```python
from build123d import *

# Parameters (mm, degrees)
SKETCH1_R           = 3.429
SKETCH1_R_2         = 2.54
BOSS_EXTRUDE1_DEPTH = 3.2004
SKETCH2_R           = 1.7272
CUT_EXTRUDE1_DEPTH  = 3.2004
SKETCH5_R           = 1.7272
SKETCH5_W           = 40.894
SKETCH5_H           = 20.32
CUT_EXTRUDE3_DEPTH  = 4.2004
CUT_EXTRUDE4_DEPTH  = 3.2004
SKETCH8_R           = 1.7272
CUT_EXTRUDE6_DEPTH  = 3.2004
SKETCH9_R           = 2.54
CUT_EXTRUDE7_DEPTH  = 3.2004
CUT_EXTRUDE8_DEPTH  = 3.2004
FILLET1_R           = 5.08
SKETCH12_R          = 2.159
CUT_EXTRUDE10_DEPTH = 3.2004
SKETCH13_R          = 13.885201093
CUT_EXTRUDE11_DEPTH = 3.2004
SKETCH14_R          = 3.175
CUT_EXTRUDE12_DEPTH = 3.2004


with BuildPart() as part:
    # Sketch1 → Boss-Extrude1 (new body)
    with BuildSketch(Plane.XY):
        with BuildLine():
            Line((0, 0), (120.015, 0))
            ThreePointArc((120.015, 0), (130.351788396, 3.075697789), (137.325636158, 11.302152592))
            Line((137.325636158, 11.302152592), (155.2575, 52.11572))
            ThreePointArc((155.2575, 52.11572), (157.086103359, 70.33575546), (147.862829498, 86.154880014))
            ThreePointArc((147.862829498, 86.154880014), (60.0075, 119.675648405), (-27.847829498, 86.154880014))
            ThreePointArc((-27.847829498, 86.154880014), (-37.071103359, 70.33575546), (-35.2425, 52.11572))
            Line((-35.2425, 52.11572), (-17.310636158, 11.302152592))
            ThreePointArc((-17.310636158, 11.302152592), (-10.336788396, 3.075697789), (0, 0))
        make_face()
        with Locations((120.015, 18.90776)):
            Circle(SKETCH1_R, mode=Mode.SUBTRACT)
        with Locations((0, 18.90776)):
            Circle(SKETCH1_R, mode=Mode.SUBTRACT)
        with Locations((19.734727639, 25.566426996)):
            Circle(SKETCH1_R_2, mode=Mode.SUBTRACT)
    extrude(amount=BOSS_EXTRUDE1_DEPTH)

    # Sketch2 → Cut-Extrude1 (cut)
    with BuildSketch(Plane(origin=(0, 0, 0), x_dir=(-1, 0, 0), z_dir=(0, 0, -1))):
        with Locations((-92.0115, 52.11572)):
            Circle(SKETCH2_R)
        with Locations((-76.0095, 52.11572)):
            Circle(SKETCH2_R)
        with Locations((-44.0055, 52.11572)):
            Circle(SKETCH2_R)
        with Locations((-28.0035, 52.11572)):
            Circle(SKETCH2_R)
    extrude(amount=-CUT_EXTRUDE1_DEPTH, mode=Mode.SUBTRACT)

    # Sketch5 → Cut-Extrude3 (cut, through all)
    with BuildSketch(Plane(origin=(0, 0, 0), x_dir=(-1, 0, 0), z_dir=(0, 0, -1))):
        with Locations((-79.746999972, 23.90776)):
            Circle(SKETCH5_R)
        with Locations((-29.246999972, 13.90776)):
            Circle(SKETCH5_R)
        with Locations((-29.246999972, 23.90776)):
            Circle(SKETCH5_R)
        with Locations((-79.746999972, 13.90776)):
            Circle(SKETCH5_R)
        with Locations((-92.322240346, 23.90776)):
            Circle(SKETCH5_R)
        with Locations((-92.322240346, 13.90776)):
            Circle(SKETCH5_R)
        with Locations((-54.496999972, 18.90776)):
            Rectangle(SKETCH5_W, SKETCH5_H)
    extrude(amount=-CUT_EXTRUDE3_DEPTH, mode=Mode.SUBTRACT)

    # Sketch6 → Cut-Extrude4 (cut)
    with BuildSketch(Plane.XY.offset(3.2004)):
        with BuildLine():
            Line((29.985999972, 19.92376), (34.049999972, 19.92376))
            Line((34.049999972, 19.92376), (34.049999972, 17.89176))
            Line((34.049999972, 17.89176), (29.985999972, 17.89176))
            ThreePointArc((29.985999972, 17.89176), (28.969999972, 18.90776), (29.985999972, 19.92376))
        make_face()
        with BuildLine():
            Line((74.943999972, 19.92376), (79.007999972, 19.92376))
            ThreePointArc((79.007999972, 19.92376), (80.023999972, 18.90776), (79.007999972, 17.89176))
            Line((79.007999972, 17.89176), (74.943999972, 17.89176))
            Line((74.943999972, 17.89176), (74.943999972, 19.92376))
        make_face()
    extrude(amount=-CUT_EXTRUDE4_DEPTH, mode=Mode.SUBTRACT)

    # Sketch8 → Cut-Extrude6 (cut)
    with BuildSketch(Plane.XY.offset(3.2004)):
        with Locations((21.9075, 3.81)):
            Circle(SKETCH8_R)
        with Locations((60.0075, 3.81)):
            Circle(SKETCH8_R)
        with Locations((98.1075, 3.81)):
            Circle(SKETCH8_R)
    extrude(amount=-CUT_EXTRUDE6_DEPTH, mode=Mode.SUBTRACT)

    # Sketch9 → Cut-Extrude7 (cut)
    with BuildSketch(Plane.XY.offset(3.2004)):
        with Locations((126.474462556, 80.535782848)):
            Circle(SKETCH9_R)
    extrude(amount=-CUT_EXTRUDE7_DEPTH, mode=Mode.SUBTRACT)

    # Sketch10 → Cut-Extrude8 (cut)
    with BuildSketch(Plane.XY.offset(3.2004)):
        with BuildLine():
            Line((25.781769816, 115.1574819), (47.097944047, 102.932721584))
            Line((47.097944047, 102.932721584), (88.071918158, 94.816913209))
            Line((88.071918158, 94.816913209), (110.992429932, 109.422556159))
            ThreePointArc((110.992429932, 109.422556159), (68.86413804, 119.377946373), (25.781769816, 115.1574819))
        make_face()
    extrude(amount=-CUT_EXTRUDE8_DEPTH, mode=Mode.SUBTRACT)

    # Fillet1
    fillet1_edges = [part.edges().sort_by_distance(p)[0] for p in [
        (110.992429932, 109.422556159, 1.6002),
        (25.781769816, 115.1574819, 1.6002),
    ]]
    fillet(fillet1_edges, radius=FILLET1_R)

    # Sketch12 → Cut-Extrude10 (cut)
    with BuildSketch(Plane.XY.offset(3.2004)):
        with Locations((24.003, 70.53072)):
            Circle(SKETCH12_R)
        with Locations((32.004, 70.53072)):
            Circle(SKETCH12_R)
        with BuildLine():
            Line((21.6535, 80.05572), (34.3535, 80.05572))
            ThreePointArc((34.3535, 80.05572), (37.5285, 76.88072), (34.3535, 73.70572))
            Line((34.3535, 73.70572), (21.6535, 73.70572))
            ThreePointArc((21.6535, 73.70572), (18.4785, 76.88072), (21.6535, 80.05572))
        make_face()
    extrude(amount=-CUT_EXTRUDE10_DEPTH, mode=Mode.SUBTRACT)

    # Sketch13 → Cut-Extrude11 (cut)
    with BuildSketch(Plane.XY.offset(3.2004)):
        with Locations((49.53, 18.90776)):
            Circle(SKETCH13_R)
    extrude(amount=-CUT_EXTRUDE11_DEPTH, mode=Mode.SUBTRACT)

    # Sketch14 → Cut-Extrude12 (cut)
    with BuildSketch(Plane.XY.offset(3.2004)):
        with Locations((78.9305, 67.99072)):
            Circle(SKETCH14_R)
        with Locations((104.3305, 67.99072)):
            Circle(SKETCH14_R)
    extrude(amount=-CUT_EXTRUDE12_DEPTH, mode=Mode.SUBTRACT)


solid = part.part
```
Input: part model. Units: mm. Frame: model coordinates. A direction names the side the tool comes from. Give positions to 0.01 mm unless a question says otherwise; leave off trailing zeros. Write each loop counter-clockwise with the first axis right and the second up, starting at its lowest first coordinate (ties: lowest second). Pieces come first, ordered by that corner, then holes. Notation, with made-up numbers: (68.25, -31.75) - (104.25, -31.75) arc R17 cw to (104.25, -0.75) - close; hole circle Ø5 at (88, 32.25). An arc over 180 degrees is marked (long way). Write item = value, one per line. Start each with the question number.
1) Cut plane C-C (y = 46.5). Return loops of the section in (x, z).
2) Draft query along X for faces 4 (the face through (130.22, 2.99, 1.58)), 5 (the face through (98.253, 101.304, 1.623)), 6 (the face through (93.693, 12.857, 1.578)), 7 (the face through (-26.4, 31.99, 1.58)). Return one class per face: pulls with the +X half, pulls with the -X half, needs draft (parallel to the pull), parting line crosses it, or undercut.
3) Material intervals for L1, parallel to X at y = 51.5, z = 0.85; L2, parallel to Y at x = 93, z = 0.3; L3, parallel to X at y = 107, z = 3, sorted ascending. Write a range as [from, to].
4) Reachability of faces 1 (the face through (157.14, 70.08, 1.58)), 2 (the face through (37.224, 108.595, 1.623)), 3 (the face through (49.384, 5.023, 1.623)) from +Z, -Z, +X, -X, +Y, -Y: full face, straight path, thin tool, end or side. Return the list, or none.
5) Cut plane A-A (z = 2.65). Give the number of separate pieces and of enclosed holes in the cut face, and give its area (3 significant figures).
6) Pin query (flat end, axial travel): pin 1 (10 mm diameter, centred on x = 104.33, y = 67.99, fed in from +Z); pin 2 (3 mm diameter, centred on x = 79.75, y = 13.91, fed in from -Z); pin 3 (1 mm diameter, centred on y = 100.5, z = 1.5, fed in from -X). Return the tip coordinate at first contact, or that it passes through.
7) Cut plane B-B (x = 9). Return loops of the section in (y, z).
Answers follow:
q1.outline = (-32.78, 0) - (152.79, 0) - (152.79, 3.2) - (-32.78, 3.2) - close
q2.face_4 = pulls with the +X half
q2.face_5 = undercut
q2.face_6 = undercut
q2.face_7 = pulls with the -X half
q3.L1 = [-34.97, 26.39], [29.62, 42.39], [45.62, 74.4], [77.62, 90.4], [93.63, 154.99]
q3.L2 = [0, 12.32], [15.5, 22.32], [25.5, 50.7], [53.53, 97.96]
q3.L3 = [3.59, 40.01], [107.19, 116.43]
q4.face_1 = +Z, -Z, +X
q4.face_2 = +Z, -Z, +Y
q4.face_3 = +Z, -Z
q5.separate_pieces = 1
q5.enclosed_holes = 23
q5.area = 16,600 mm^2
q6.pin_1 = 3.2
q6.pin_2 = through
q6.pin_3 = -9.3
q7.outline = (0, 0) - (109.41, 0) - (109.41, 3.2) - (0, 3.2) - close
